Work out the finished part from the listing and answer in its coordinate system (mm). Give positions to 0.01 mm unless a question says otherwise; leave off trailing zeros. Loops run counter-clockwise (first coordinate to the right, second up) from the corner with the lowest first, then second, coordinate; pieces in that order, holes last.
```python
from build123d import *

# Parameters (mm, degrees)
F0_W     = 38.1
F0_H     = 4.7625
F0_R     = 2.301875
F1_DEPTH = 7.9375
F2_R     = 2.38125
F3_DEPTH = 25.4


with BuildPart() as f1:
    # F0 (on Top) → F1 (new body)
    with BuildSketch(Plane.XY):
        with Locations((19.05, 2.38125)):
            Rectangle(F0_W, F0_H)
        with Locations((4.7625, 2.38125)):
            Circle(F0_R, mode=Mode.SUBTRACT)
        with Locations((19.05, 2.38125)):
            Circle(F0_R, mode=Mode.SUBTRACT)
        with Locations((33.3375, 2.38125)):
            Circle(F0_R, mode=Mode.SUBTRACT)
    extrude(amount=F1_DEPTH)

    # F2 (on face) → F3 (cut)
    with BuildSketch(Plane.XZ):
        with Locations((28.575, 3.96875)):
            Circle(F2_R)
        with Locations((9.525, 3.96875)):
            Circle(F2_R)
    extrude(amount=-F3_DEPTH, mode=Mode.SUBTRACT)


solid = f1.part
```
Q1. Section D-D on x = 32.5 is taken. Give the vertices of the cut face in (y, z), plus the area to 3 significant figures.
Q2. Section A-A on x = 19.05 is taken. Give the vertices of the cut face in (y, z), plus the area to 3 significant figures.
Q3. Consider line 1 along X through (y, z) = (3.6, 3.25); line 2 along X through (y, z) = (1.65, 5.5); line 3 along X through (y, z) = (2.5, 0.5). Determine where each line is inside the solid, lowest interval first.
Q4. Determine the mould class of faces 1 (the face through (26.196, 2.348, 4.073)), 2 (the face through (23, 2, 7.938)), 3 (the face through (38.1, 2, 4)) for opening direction X: +X half, -X half, draft (parallel to the pull), parting line (faces both ways), or undercut.
Q5. Section B-B on z = 3 is taken. Give the vertices of the cut face in (x, y), plus the area to 3 significant figures.
Q6. Section C-C on y = 1.3 is taken. Give the vertices of the cut face in (x, z) (1 decimal).
Check result:
1. outline: (0, 0) - (0.24, 0) - (0.24, 7.94) - (0, 7.94) - close; (4.53, 0) - (4.76, 0) - (4.76, 7.94) - (4.53, 7.94) - close
1. area: 3.76 mm2
2. outline: (0, 0) - (0.08, 0) - (0.08, 7.94) - (0, 7.94) - close; (4.68, 0) - (4.76, 0) - (4.76, 7.94) - (4.68, 7.94) - close
2. area: 1.26 mm2
3. line 1: x = 0 to 2.81, 6.72 to 7.25, 11.8 to 17.1, 21 to 26.3, 30.85 to 31.38, 35.29 to 38.1
3. line 2: x = 0 to 2.58, 6.95 to 7.7, 11.35 to 16.87, 21.23 to 26.75, 30.4 to 31.15, 35.52 to 38.1
3. line 3: x = 0 to 2.46, 7.06 to 16.75, 21.35 to 31.04, 35.64 to 38.1
4. face 1: undercut
4. face 2: draft
4. face 3: +X half
5. outline: (0, 0) - (7.35, 0) - (7.35, 4.76) - (0, 4.76) - close; (11.7, 0) - (26.4, 0) - (26.4, 4.76) - (11.7, 4.76) - close; (30.75, 0) - (38.1, 0) - (38.1, 4.76) - (30.75, 4.76) - close; hole circle Ø4.6 at (4.76, 2.38); hole circle Ø4.6 at (19.05, 2.38); hole circle Ø4.6 at (33.34, 2.38)
5. area: 90.1 mm2
6. outline: (0, 0) - (2.7, 0) - (2.7, 7.9) - (0, 7.9) - close; (6.8, 0) - (17, 0) - (17, 7.9) - (6.8, 7.9) - close; (21.1, 0) - (31.3, 0) - (31.3, 7.9) - (21.1, 7.9) - close; (35.4, 0) - (38.1, 0) - (38.1, 7.9) - (35.4, 7.9) - close; hole circle Ø4.8 at (9.5, 4); hole circle Ø4.8 at (28.6, 4)
